The listing builds one solid part. Answer for the finished solid, in the listing's coordinates (mm). A direction names the side the tool comes from. Round coordinates to 2 decimals unless told otherwise and drop trailing zeros. Write each loop counter-clockwise with the first axis right and the second up, starting at its lowest first coordinate (ties: lowest second). Pieces come first, ordered by that corner, then holes. Notation, with made-up numbers: M 12,-6.5 L 58,-6.5 A18 ccw 58,25.5 Z; hole C -30,69.5 d7. An arc over 180 degrees is marked long. Put each result on its own line as item: value. Start each with the question number.
```python
from build123d import *

# Parameters (mm, degrees)
F1_DEPTH = 1500
F2_R     = 1.5
F4_D     = 18


with BuildPart() as f1:
    # F0 (on Front) → F1 (new body)
    with BuildSketch(Plane.XZ):
        Polygon((5.458542, 61.221596), (6.958542, 61.057889), (6.958542, 76.057889), (-59.041458, 76.057889), (-59.041458, -73.942111), (6.958542, -73.942111), (6.958542, -58.942111), (5.458542, -58.942111), (5.458542, -72.442111), (-57.541458, -72.442111), (-57.541458, 74.557889), (5.458542, 74.557889), align=None)
    extrude(amount=-F1_DEPTH)

    # F2
    f2_edges = [f1.edges().sort_by_distance(p)[0] for p in [
        (-59.041458, 750, 76.057889),
        (6.958542, 750, 76.057889),
        (6.958542, 750, -73.942111),
        (-59.041458, 750, -73.942111),
    ]]
    fillet(f2_edges, radius=F2_R)

    # F4 (through all)
    with Locations(Plane.YZ.offset(-57.541458)):
        with Locations((32, 34.057889), (102, 34.057889), (31.999985, -32.942111), (102, -32.942111), (1468, 34.057889), (1398, 34.057889), (1398, -32.942111), (1468, -32.942111)):
            Hole(F4_D / 2)


solid = f1.part
```
Item 1: Section A-A (x = -21.5) is taken. Give the vertices of the cut face in (y, z), and give its area (3 significant figures).
Item 2: Flat-ended cylindrical pins translate along their axes: pin 1 (14.5 mm diameter, centred on y = 102, z = 34.06, fed in from +X); pin 2 (6 mm diameter, centred on y = 1347.5, z = -19.5, fed in from +X). Find the tip coordinate at first contact, or state that the pin passes through.
Item 3: Section B-B (y = 657.5) is taken. Give the vertices of the cut face in (x, z).
Item 4: Determine the mould class of faces 1 (the flat face through (-59.041, 740, 2)), 2 (the flat face through (-58, 1500, 1)), 3 (the flat face through (-26, 740, -72.442)) for opening direction X: released by +X, released by -X, zero draft, split by the parting line, or undercut.
Item 5: Consider line 1 along Z through (x, y) = (-58.05, 1468); line 2 along Z through (x, y) = (-24, 260.5); line 3 along X through (y, z) = (1433, -62). Determine where each line is inside the solid, lowest interval first. Write a range as [from, to].
Item 6: Which of the six approach directions +Z, -Z, +X, -X, +Y, -Y give full straight-line access (tool end or side, diameter ignored) to faces 4 (the flat face through (-26, 740, 74.558)), 5 (the flat face through (-58, 0, 1))?
Output values:
1. outline: M 0,-73.94 L 1500,-73.94 L 1500,-72.44 L 0,-72.44 Z; M 0,74.56 L 1500,74.56 L 1500,76.06 L 0,76.06 Z
1. area: 4,500 mm^2
2. pin 1: passes through
2. pin 2: stops at x = -57.54
3. outline: M -59.04,-72.44 A1.5 ccw -57.54,-73.94 L 5.46,-73.94 A1.5 ccw 6.96,-72.44 L 6.96,-58.94 L 5.46,-58.94 L 5.46,-72.44 L -57.54,-72.44 L -57.54,74.56 L 5.46,74.56 L 5.46,61.22 L 6.96,61.06 L 6.96,74.56 A1.5 ccw 5.46,76.06 L -57.54,76.06 A1.5 ccw -59.04,74.56 Z
4. face 1: released by -X
4. face 2: zero draft
4. face 3: undercut
5. line 1: z = [-73.85, -41.94], [-23.94, 25.06], [43.06, 75.97]
5. line 2: z = [-73.94, -72.44], [74.56, 76.06]
5. line 3: x = [-59.04, -57.54], [5.46, 6.96]
6. face 4: +Y, -Y
6. face 5: +Z, -Z, +X, -X, -Y
